Work out the finished part from the listing and answer in its coordinate system (mm). A direction names the side the tool comes from. Coordinates: 2 decimals unless noted, no trailing zeros. Order: outer loops, then holes, each group sorted by start corner. A loop starts at its lowest first (then second) coordinate and runs counter-clockwise, first axis right, second up.
```python
from build123d import *

# Parameters (mm, degrees)
OUTER_FRAME_EXTRUDE_DEPTH      = 4
OUTER_FRAME_EXTRUDE_DEPTH_BACK = 2
OUTSIDE_FRAME_W                = 18.2
OUTSIDE_FRAME_H                = 18.2
OUTSIDE_FRAME_W_2              = 14.2
OUTSIDE_FRAME_H_2              = 14.2
HOTSWAP_BASE_W                 = 18.2
HOTSWAP_BASE_H                 = 11.5
HOTSWAP_BASE_BLOCK_DEPTH       = 4
CUT_EXTRUDE4_DEPTH             = 16.15321748
CUT_EXTRUDE4_DEPTH_BACK        = 16.15321748
SKETCH1_W                      = 2
SKETCH1_H                      = 6.7
CUT_EXTRUDE1_DEPTH             = 4
SWITCH_PIN_HOLES_R             = 2
SWITCH_PIN_HOLES_R_2           = 1.25
SWITCH_HOLES_DEPTH             = 3.6
CUT_EXTRUDE3_REACH             = 17.153
HOTSWAP_HOLES_R                = 1.6
CHAMFER1_SIZE                  = 2
CHAMFER2_SIZE                  = 4
FILLET1_R                      = 0.35
CHAMFER3_SIZE                  = 0.75


# Some blends are built 0.0001 mm under size
with BuildPart() as part:
    # Outside Frame → Outer Frame Extrude (new, two sides: drawn at the far end of the back side and taken through both)
    with BuildSketch(Plane.XY.offset(-4).offset(-OUTER_FRAME_EXTRUDE_DEPTH_BACK)):
        Rectangle(OUTSIDE_FRAME_W, OUTSIDE_FRAME_H)
        Rectangle(OUTSIDE_FRAME_W_2, OUTSIDE_FRAME_H_2, mode=Mode.SUBTRACT)
    extrude(amount=OUTER_FRAME_EXTRUDE_DEPTH + OUTER_FRAME_EXTRUDE_DEPTH_BACK)

    # Hotswap Base → Hotswap Base Block (add)
    with BuildSketch(Plane.XY.offset(-4)):
        with Locations((0, -3.35)):
            Rectangle(HOTSWAP_BASE_W, HOTSWAP_BASE_H)
    extrude(amount=-HOTSWAP_BASE_BLOCK_DEPTH)

    # Sketch1 → Cut-Extrude4 (cut, two sides: drawn at the far end of the back side and taken through both)
    with BuildSketch(Plane(origin=(0, 0, 0), x_dir=(0, 0, -1), z_dir=(1, 0, 0)).offset(-CUT_EXTRUDE4_DEPTH_BACK)):
        with Locations((5, 5.75)):
            Rectangle(SKETCH1_W, SKETCH1_H)
    extrude(amount=CUT_EXTRUDE4_DEPTH + CUT_EXTRUDE4_DEPTH_BACK, mode=Mode.SUBTRACT)

    # Hotswap Well → Cut-Extrude1 (cut)
    with BuildSketch(Plane(origin=(0, 0, -6), x_dir=(-1, 0, 0), z_dir=(0, 0, -1))):
        with BuildLine():
            Line((-10, -1.1), (-2.355843798, -1.1))
            ThreePointArc((-2.355843798, -1.1), (-1.396424004, -2.19317122), (0, -2.6))
            Line((0, -2.6), (5, -2.6))
            Line((5, -2.6), (5, -3.35))
            Line((5, -3.35), (10, -3.35))
            Line((10, -3.35), (10, -6.9))
            Line((10, -6.9), (-6, -6.9))
            Line((-6, -6.9), (-6, -4.1))
            Line((-6, -4.1), (-10, -4.1))
            Line((-10, -4.1), (-10, -1.1))
        make_face()
    extrude(amount=CUT_EXTRUDE1_DEPTH, mode=Mode.SUBTRACT)

    # Switch Pin Holes → Switch Holes (cut)
    with BuildSketch(Plane.XY.offset(-4)):
        Circle(SWITCH_PIN_HOLES_R)
        with Locations((-5, 0)):
            Circle(SWITCH_PIN_HOLES_R_2)
        with Locations((5, 0)):
            Circle(SWITCH_PIN_HOLES_R_2)
    extrude(amount=-SWITCH_HOLES_DEPTH, mode=Mode.SUBTRACT)

    # Cut-Extrude3: up to this face of the body (flat: up to its plane)
    cut_extrude3_end = Plane(part.part.faces().sort_by_distance((5, 0.029137252, -7.6))[0])
    # Hotswap Holes → Cut-Extrude3 (cut, up to the picked face)
    with BuildSketch(Plane.XY, mode=Mode.PRIVATE) as cut_extrude3_sk1:
        with Locations((-2.560136595, -4.965291588)):
            Circle(HOTSWAP_HOLES_R)
    cut_extrude3_tool1 = split(extrude(cut_extrude3_sk1.sketch, amount=-CUT_EXTRUDE3_REACH, mode=Mode.PRIVATE), bisect_by=cut_extrude3_end, keep=Keep.BOTH, mode=Mode.PRIVATE)
    # Hotswap Holes → Cut-Extrude3 (cut, up to the picked face)
    with BuildSketch(Plane.XY, mode=Mode.PRIVATE) as cut_extrude3_sk2:
        with BuildLine():
            Line((3.930924016, 0.647747281), (2.46548889, -1.77088348))
            ThreePointArc((2.46548889, -1.77088348), (3.179147124, -4.059894044), (5.3631684, -3.070485887))
            Line((5.3631684, -3.070485887), (6.194736133, -0.367567099))
            ThreePointArc((6.194736133, -0.367567099), (5.511530489, 1.140542222), (3.930924016, 0.647747281))
        make_face()
    cut_extrude3_tool2 = split(extrude(cut_extrude3_sk2.sketch, amount=-CUT_EXTRUDE3_REACH, mode=Mode.PRIVATE), bisect_by=cut_extrude3_end, keep=Keep.BOTH, mode=Mode.PRIVATE)
    add(cut_extrude3_tool1.solids().sort_by(Axis((-2.560137, -4.965292, 0), (0, 0, -1)))[0], mode=Mode.SUBTRACT)
    add(cut_extrude3_tool2.solids().sort_by(Axis((4.301523, -1.557372, 0), (0, 0, -1)))[0], mode=Mode.SUBTRACT)

    # Chamfer1
    chamfer1_edges = [part.edges().sort_by_distance(p)[0] for p in [
        (9.1, -4.1, -7),
        (-9.1, -6.9, -7),
        (-9.1, -3.35, -7),
        (9.1, -1.1, -7),
    ]]
    chamfer(chamfer1_edges, length=CHAMFER1_SIZE)

    # Chamfer2
    chamfer2_edges = [part.edges().sort_by_distance(p)[0] for p in [
        (-8.1, 2.4, -4),
        (8.1, 2.4, -4),
    ]]
    chamfer(chamfer2_edges, length=CHAMFER2_SIZE - 0.0001)  # a hair under: the kernel refuses the full size

    # Fillet1
    fillet1_edges = [part.edges().sort_by_distance(p)[0] for p in [
        (6, -4.1, -7),
        (-5, -3.35, -7),
        (-5, -2.6, -7),
        (6, -6.9, -7),
        (2.355843798, -1.1, -7),
    ]]
    fillet(fillet1_edges, radius=FILLET1_R)

    # Chamfer3
    # the kernel refuses this chamfer: 0.75 mm, written as the material it takes off along each edge
    with BuildSketch(Plane(origin=(9.1, 4.328762241, -8), x_dir=(-0.9996219169112965, 0, -0.02749587661058676), z_dir=(0, -1, 0))) as chamfer3_piece_1:
        Polygon((CHAMFER3_SIZE * 0.999621916911, -CHAMFER3_SIZE * 0.0274958766106), (-CHAMFER3_SIZE * 0.0274958766106, -CHAMFER3_SIZE * 0.999621916911), (0, 0), align=None)
    extrude(amount=5.357524482, mode=Mode.SUBTRACT)
    with BuildSketch(Plane(origin=(-9.1, -3.278762241, -8), x_dir=(0.9996219169112965, 0, -0.02749587661058676), z_dir=(0, 1, 0))) as chamfer3_piece_2:
        Polygon((CHAMFER3_SIZE * 0.999621916911, -CHAMFER3_SIZE * 0.0274958766106), (-CHAMFER3_SIZE * 0.0274958766106, -CHAMFER3_SIZE * 0.999621916911), (0, 0), align=None)
    extrude(amount=7.607524482, mode=Mode.SUBTRACT)
    with BuildSketch(Plane(origin=(-9.1, -11.028762241, -8), x_dir=(-0.027495876610586768, 0, 0.9996219169112968), z_dir=(0, 1, 0))) as chamfer3_piece_3:
        Polygon((CHAMFER3_SIZE * 0.999621916911, CHAMFER3_SIZE * 0.0274958766106), (-CHAMFER3_SIZE * 0.0274958766106, CHAMFER3_SIZE * 0.999621916911), (0, 0), align=None)
    extrude(amount=4.057524482, mode=Mode.SUBTRACT)
    with BuildSketch(Plane(origin=(9.1, -4.171237759, -8), x_dir=(0.027495876610586768, 0, 0.9996219169112968), z_dir=(0, -1, 0))) as chamfer3_piece_4:
        Polygon((CHAMFER3_SIZE * 0.999621916911, CHAMFER3_SIZE * 0.0274958766106), (-CHAMFER3_SIZE * 0.0274958766106, CHAMFER3_SIZE * 0.999621916911), (0, 0), align=None)
    extrude(amount=6.857524482, mode=Mode.SUBTRACT)
    with BuildSketch(Plane(origin=(11.028762241, -9.1, -8), x_dir=(0, -0.027495876610586768, 0.9996219169112968), z_dir=(-1, 0, 0))) as chamfer3_piece_5:
        Polygon((CHAMFER3_SIZE * 0.999621916911, CHAMFER3_SIZE * 0.0274958766106), (-CHAMFER3_SIZE * 0.0274958766106, CHAMFER3_SIZE * 0.999621916911), (0, 0), align=None)
    extrude(amount=22.057524482, mode=Mode.SUBTRACT)
    with BuildSketch(Plane(origin=(-11.028762241, 2.4, -8), x_dir=(0, -0.9996219169112968, -0.027495876610586775), z_dir=(1, 0, 0))) as chamfer3_piece_6_section:
        Polygon((CHAMFER3_SIZE * 0.999621916911, -CHAMFER3_SIZE * 0.0274958766106), (-CHAMFER3_SIZE * 0.0274958766106, -CHAMFER3_SIZE * 0.999621916911), (0, 0), align=None)
    chamfer3_piece_6 = extrude(amount=22.057524482, mode=Mode.PRIVATE)
    chamfer3_piece_6 = split(chamfer3_piece_6, bisect_by=Plane(origin=(7.1, 2.149999996, -7.749999996), z_dir=(-1, 0, 0)), keep=Keep.TOP, mode=Mode.PRIVATE)
    chamfer3_piece_6 = split(chamfer3_piece_6, bisect_by=Plane(origin=(-7.1, 2.149999996, -7.749999996), z_dir=(1, 0, 0)), keep=Keep.TOP, mode=Mode.PRIVATE)
    add(chamfer3_piece_6, mode=Mode.SUBTRACT)
    with BuildSketch(Plane(origin=(9.1, 7.76374086, -2.63615914), x_dir=(0.02749587661058679, -0.7068394360706739, 0.706839436070673), z_dir=(0, -0.7071067811865471, -0.7071067811865479))) as chamfer3_piece_7_section:
        Polygon((CHAMFER3_SIZE * 0.999621916911, CHAMFER3_SIZE * 0.0274958766106), (-CHAMFER3_SIZE * 0.0274958766106, CHAMFER3_SIZE * 0.999621916911), (0, 0), align=None)
    chamfer3_piece_7 = extrude(amount=9.51423731, mode=Mode.PRIVATE)
    chamfer3_piece_7 = split(chamfer3_piece_7, bisect_by=Plane(origin=(8.843939938, 4.231743527, -4), z_dir=(0, 0, -1)), keep=Keep.TOP, mode=Mode.PRIVATE)
    add(chamfer3_piece_7, mode=Mode.SUBTRACT)
    with BuildSketch(Plane(origin=(-9.1, 7.76374086, -2.63615914), x_dir=(-0.027495876610586768, -0.7068394360706739, 0.706839436070673), z_dir=(0, -0.7071067811865471, -0.7071067811865479))) as chamfer3_piece_8_section:
        Polygon((CHAMFER3_SIZE * 0.999621916911, -CHAMFER3_SIZE * 0.0274958766106), (-CHAMFER3_SIZE * 0.0274958766106, -CHAMFER3_SIZE * 0.999621916911), (0, 0), align=None)
    chamfer3_piece_8 = extrude(amount=9.51423731, mode=Mode.PRIVATE)
    chamfer3_piece_8 = split(chamfer3_piece_8, bisect_by=Plane(origin=(-8.843939938, 4.231743527, -4), z_dir=(0, 0, -1)), keep=Keep.TOP, mode=Mode.PRIVATE)
    add(chamfer3_piece_8, mode=Mode.SUBTRACT)

    # Split1
    split(bisect_by=Plane.XY.offset(-4), keep=Keep.BOTTOM)


solid = part.part
```
1. The part is cut by section D-D (x = 0.5). Determine the outline of the cut face in (y, z).
2. The mould has two halves that part along X. Classify faces 1 (the flat face through (0, -3, -4)), 2 (the flat face through (-8.09, -2.36, -7.01)), 3 (the flat face through (0, 0, -7.6)): released by +X, released by -X, zero draft, split by the parting line, or undercut.
3. Consider probe 1 along Y at (x, z) = (0, -6.25); probe 2 along Y at (x, z) = (0, -5.55); probe 3 along Y at (x, z) = (-1.75, -7.5). Determine where each line is inside the solid, lowest interval first.
4. For faces 4 (the flat face through (-6, -3.35, -7)), 5 (the flat face through (5, 0, -7.6)), 6 (the flat face through (-1, -6.9, -7)), 7 (the flat face through (0, -4, -6)), 8 (the flat face through (-2, -2.6, -7)), determine the directions among +Z, -Z, +X, -X, +Y, -Y from which every point of the face is accessible in a straight line to the end or side of a thin tool.
5. The part is cut by section C-C (y = 4.25). Determine the outline of the cut face in (x, z).
6. A flat-ended cylindrical pin translates along its axis: pin 1 (1.5 mm diameter, centred on x = -4.5, z = -7.5, fed in from +Y). Find the tip coordinate at first contact, or state that the pin passes through.
7. The part is cut by section B-B (z = -6.9). Count the separate pieces of the cut face and the enclosed holes in it, plus the area to 3 significant figures.
Worked out:
1. outline: (-9.1, -7.25) - (-8.35, -8) - (-6.9, -8) - (-6.9, -6) - (-2.55, -6) - (-2.55, -8) - (1.65, -8) - (2.4, -7.25) - (2.4, -4) - (1.94, -4) - (1.94, -7.6) - (-1.94, -7.6) - (-1.94, -4) - (-9.1, -4) - close
2. face 1: zero draft
2. face 2: released by -X
2. face 3: undercut
3. probe 1: y = -9.1 to -6.9, -2.6 to -2, 2 to 2.4
3. probe 2: y = -9.1 to -2, 2 to 2.4
3. probe 3: y = -8.85 to -6.9, -2.6 to -0.97, 0.97 to 2.15
4. face 4: -Z, +X, -X
4. face 5: +Z
4. face 6: -Z, -X
4. face 7: -Z
4. face 8: -Z, +X
5. outline: (-9.1, -5.09) - (-8.35, -6.15) - (-7.1, -6.15) - (-7.1, -4) - (-9.1, -4) - close; (7.1, -6.15) - (8.35, -6.15) - (9.1, -5.09) - (9.1, -4) - (7.1, -4) - close
6. pin 1: stops at y = 2.4
7. separate pieces: 2
7. enclosed holes: 2
7. area: 104 mm2
